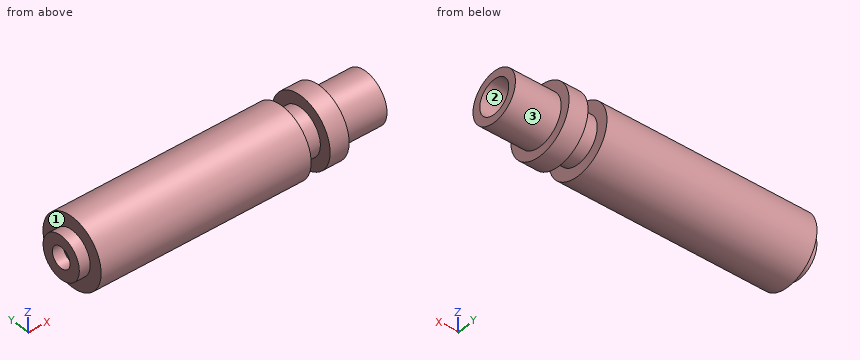
```python
from build123d import *

# Parameters (mm, degrees)
SKETCH1_R           = 15.07617
BOSS_EXTRUDE1_DEPTH = 108.4446395
SKETCH2_R           = 9.3853
SKETCH2_R_2         = 4.5847
BOSS_EXTRUDE2_DEPTH = 4.7498
SKETCH3_R           = 7.5
CUT_EXTRUDE1_DEPTH  = 18.75
BOSS_EXTRUDE3_START = 20
SKETCH4_R           = 11
SKETCH4_R_2         = 7.5
BOSS_EXTRUDE3_DEPTH = 20
CUT_EXTRUDE4_START  = -8.3023864
SKETCH5_R           = 15.07617
SKETCH5_R_2         = 10
CUT_EXTRUDE4_DEPTH  = 8.3023864


with BuildPart() as part:
    # Sketch1 → Boss-Extrude1 (new body)
    with BuildSketch(Plane(origin=(0, 0, 0), x_dir=(0, 0, -1), z_dir=(1, 0, 0))):
        Circle(SKETCH1_R)
    extrude(amount=BOSS_EXTRUDE1_DEPTH)

    # Sketch2 → Boss-Extrude2 (add)
    with BuildSketch(Plane.ZY):
        with Locations(Location((0, 0, 0), (0, 0, 180))):
            Circle(SKETCH2_R)
        Circle(SKETCH2_R_2, mode=Mode.SUBTRACT)
    extrude(amount=BOSS_EXTRUDE2_DEPTH)

    # Sketch3 → Cut-Extrude1 (cut)
    with BuildSketch(Plane(origin=(108.4446395, 0, 0), x_dir=(0, 0, -1), z_dir=(1, 0, 0))):
        Circle(SKETCH3_R)
    extrude(amount=-CUT_EXTRUDE1_DEPTH, mode=Mode.SUBTRACT)

    # Sketch4 → Boss-Extrude3 (add)
    with BuildSketch(Plane(origin=(108.4446395, 0, 0), x_dir=(0, 0, -1), z_dir=(1, 0, 0)).offset(BOSS_EXTRUDE3_START)):
        Circle(SKETCH4_R)
        Circle(SKETCH4_R_2, mode=Mode.SUBTRACT)
    extrude(amount=-BOSS_EXTRUDE3_DEPTH)

    # Sketch5 → Cut-Extrude4 (cut)
    with BuildSketch(Plane(origin=(100.1422531, 0, 0), x_dir=(0, 0, -1), z_dir=(1, 0, 0)).offset(CUT_EXTRUDE4_START)):
        Circle(SKETCH5_R)
        Circle(SKETCH5_R_2, mode=Mode.SUBTRACT)
    extrude(amount=CUT_EXTRUDE4_DEPTH, mode=Mode.SUBTRACT)


solid = part.part
```
Verification items for the finished model (mm, model axes). Face numbers are marked on the shaded views. Coordinates: 2 decimals unless noted, no trailing zeros. Write each loop counter-clockwise with the first axis right and the second up, starting at its lowest first coordinate (ties: lowest second). Pieces come first, ordered by that corner, then holes. Notation, with made-up numbers: (22.25, 53) - (53.25, 53) arc R22 ccw to (53.25, 74) - close; hole circle Ø6 at (66.5, 45.5). An arc over 180 degrees is marked (long way). One line per question, with ' | ' between items. Start each with the question number.
1. Section check C-C (y = -2). Enter the section's corners in (x, z).
2. Section check D-D (x = 42.5). Enter the section's corners in (y, z).
3. Section check A-A (z = -12.5). Enter the section's corners in (x, y), plus the area to 3 significant figures.
4. Draft check along Z on the marked faces 1, 2 and 3. Enter one of: released by +Z, released by -Z, zero draft, split by the parting line, or undercut.
5. Gauge pin test, flat ends, axial feed: P1, Ø12, axis at x = 30, z = 8.5, coming from the -Y side; P2, Ø1.5, axis at x = 43, z = -3.5, coming from the +Y side; P3, Ø2, axis at x = 32.5, y = 5, coming from the +Z side. Record the tip position at first contact, or that the pin passes through.
6. Section check B-B (z = 0). Enter the section's corners in (x, y), plus the area to 3 significant figures.
7. Material ranges on line 1 along X through (y, z) = (-12, 4); line 2 along Y through (x, z) = (-2.2, 0); line 3 along X through (y, z) = (5, 9), recorded low to high.
Computed values:
1) outline: (-4.75, -9.17) - (0, -9.17) - (0, -14.94) - (91.84, -14.94) - (91.84, -9.8) - (100.14, -9.8) - (100.14, -14.94) - (108.44, -14.94) - (108.44, -10.82) - (128.44, -10.82) - (128.44, -7.23) - (89.69, -7.23) - (89.69, 7.23) - (128.44, 7.23) - (128.44, 10.82) - (108.44, 10.82) - (108.44, 14.94) - (100.14, 14.94) - (100.14, 9.8) - (91.84, 9.8) - (91.84, 14.94) - (0, 14.94) - (0, 9.17) - (-4.75, 9.17) - (-4.75, 4.13) - (0, 4.13) - (0, -4.13) - (-4.75, -4.13) - close
2) outline: circle Ø30.15 at (0, 0)
3) outline: (0, -8.43) - (91.84, -8.43) - (91.84, 8.43) - (0, 8.43) - close; (100.14, -8.43) - (108.44, -8.43) - (108.44, 8.43) - (100.14, 8.43) - close | area: 1,690 mm²
4) face 1: zero draft | face 2: undercut | face 3: split by the parting line
5) P1: y = -14.87 | P2: y = 14.82 | P3: z = 14.54
6) outline: (-4.75, -9.39) - (0, -9.39) - (0, -15.08) - (91.84, -15.08) - (91.84, -10) - (100.14, -10) - (100.14, -15.08) - (108.44, -15.08) - (108.44, -11) - (128.44, -11) - (128.44, -7.5) - (89.69, -7.5) - (89.69, 7.5) - (128.44, 7.5) - (128.44, 11) - (108.44, 11) - (108.44, 15.08) - (100.14, 15.08) - (100.14, 10) - (91.84, 10) - (91.84, 15.08) - (0, 15.08) - (0, 9.39) - (-4.75, 9.39) - (-4.75, 4.58) - (0, 4.58) - (0, -4.58) - (-4.75, -4.58) - close | area: 3,090 mm²
7) line 1: 0 to 91.84, 100.14 to 108.44 | line 2: -9.39 to -4.58, 4.58 to 9.39 | line 3: 0 to 91.84, 100.14 to 128.44
